Read the model definition and answer for the solid it produces. Units are mm, in the model's axes. A direction names the side the tool comes from. Coordinates: 2 decimals unless noted, no trailing zeros. Loops run counter-clockwise (first coordinate to the right, second up) from the corner with the lowest first, then second, coordinate; pieces in that order, holes last. Notation, with made-up numbers: (-6, -4) - (3, -4) arc R11 cw to (3, 1) - close; hole circle Ø4 at (19.5, 80.5). An arc over 180 degrees is marked (long way). Use one line per item in the form item = value. Start each with the question number.
1) The mould has two halves that part along Y. Classify faces 1 (the face through (-24.43, 9.4, 1.57)), 2 (the face through (10.6, 0.11, 5.67)), 3 (the face through (-3, 0, 3)), 4 (the face through (0.11, -9.43, 9.5)): released by +Y, released by -Y, zero draft, split by the parting line, or undercut.
2) A cutting plane is placed at A-A (x = 0). Give the vertices of the cut face in (y, z).
3) Consider line 1 (X direction, y = 1, z = 3.25); line 2 (Y direction, x = 20, z = 3); line 3 (Z direction, x = -16, y = 0.5). Determine where each line is inside the solid, lowest interval first.
4) Which of the six approach directions +Z, -Z, +X, -X, +Y, -Y give full straight-line access (tool end or side, diameter ignored) to faces 5 (the face through (-9.43, -9.4, 7.61)), 6 (the face through (17, 0, 5.1)), 7 (the face through (17.58, -9.43, 4.5))?
5) A cutting plane is placed at B-B (z = 1). Give the vertices of the cut face in (x, y), and give its area (3 significant figures).
6) Each of these flat-tipped pins is pushed along its axis until it touches: P1, Ø1, axis at x = 9, z = 9, coming from the -Y side; P2, Ø3, axis at x = -1, y = 1, coming from the -Z side; P3, Ø0.8, axis at y = 1, z = 7.5, coming from the +X side; P4, Ø10.5, axis at x = 0, y = 0, coming from the +Z side. Where does it stop, or does it pass through?
7) A cutting plane is placed at D-D (z = 9.25). Give the vertices of the cut face in (x, y), and give its area (3 significant figures).
8) A cutting plane is placed at C-C (y = 0). State how many separate pieces and enclosed holes the cut face has, and give its area (3 significant figures).
from build123d import *

# Parameters (mm, degrees)
F0_W     = 50
F0_H     = 20
F0_R     = 2.25
F0_R_2   = 4
F0_R_3   = 3
F1_DEPTH = 5.1
F2_W     = 20
F2_H     = 20
F2_R     = 3
F2_R_2   = 2.25
F3_DEPTH = 2.5
F4_W     = 20
F4_H     = 20
F4_R     = 4
F5_DEPTH = 2.5
F6_R     = 2


# Not quite as in the source:
# - a feature names something its author has since deleted; it is built from what else it names


with BuildPart() as f1:
    # F0 (on Top) → F1 (new body)
    with BuildSketch(Plane.XY):
        Rectangle(F0_W, F0_H)
        with Locations((-20, 0)):
            Circle(F0_R, mode=Mode.SUBTRACT)
        Circle(F0_R_2, mode=Mode.SUBTRACT)
        with Locations((20, 0)):
            Circle(F0_R, mode=Mode.SUBTRACT)
        Circle(F0_R_2)
        Circle(F0_R_3, mode=Mode.SUBTRACT)
    extrude(amount=F1_DEPTH)

    # F2 (on face) → F3 (join)
    with BuildSketch(Plane.XY.offset(5.1)):
        Rectangle(F2_W, F2_H)
        Circle(F2_R, mode=Mode.SUBTRACT)
        Circle(F2_R)
        Circle(F2_R_2, mode=Mode.SUBTRACT)
    extrude(amount=F3_DEPTH)

    # F4 (on face) → F5 (join)
    with BuildSketch(Plane.XY.offset(7.6)):
        Rectangle(F4_W, F4_H)
        Circle(F4_R, mode=Mode.SUBTRACT)
    extrude(amount=F5_DEPTH)

    # F6
    f6_edges = [f1.edges().sort_by_distance(p)[0] for p in [
        (-25, -10, 2.55),
        (25, -10, 2.55),
        (25, 10, 2.55),
        (25, 0, 5.1),
        (17.5, -10, 5.1),
        (17.5, 10, 5.1),
        (-17.5, -10, 5.1),
        (-25, 0, 5.1),
        (-17.5, 10, 5.1),
        (-25, 10, 2.55),
        (10, -10, 7.6),
        (10, 10, 7.6),
        (-10, -10, 7.6),
        (-10, 10, 7.6),
        (10, 0, 5.1),
        (-10, 0, 5.1),
        (0, -10, 10.1),
        (-10, 0, 10.1),
        (0, 10, 10.1),
        (10, 0, 10.1),
    ]]
    fillet(f6_edges, radius=F6_R)


solid = f1.part
Found:
q1.face_1 = released by +Y
q1.face_2 = zero draft
q1.face_3 = undercut
q1.face_4 = released by -Y
q2.outline = (-10, 0) - (-3, 0) - (-3, 5.1) - (-2.25, 5.1) - (-2.25, 7.6) - (-4, 7.6) - (-4, 10.1) - (-8, 10.1) arc R2 ccw to (-10, 8.1) - close; (2.25, 5.1) - (3, 5.1) - (3, 0) - (10, 0) - (10, 8.1) arc R2 ccw to (8, 10.1) - (4, 10.1) - (4, 7.6) - (2.25, 7.6) - close
q3.line_1 = -24.99 to -22.02, -17.98 to -2.83, 2.83 to 17.98, 22.02 to 24.99
q3.line_2 = -10 to -2.25, 2.25 to 10
q3.line_3 = 0 to 5.1
q4.face_5 = +Z, -X, -Y
q4.face_6 = +Z, +X, +Y, -Y
q4.face_7 = +Z, +X, -Y
q5.outline = (-25, -8) arc R2 ccw to (-23, -10) - (23, -10) arc R2 ccw to (25, -8) - (25, 8) arc R2 ccw to (23, 10) - (-23, 10) arc R2 ccw to (-25, 8) - close; hole circle Ø4.5 at (-20, 0); hole circle Ø6 at (0, 0); hole circle Ø4.5 at (20, 0)
q5.area = 936 mm^2
q6.P1 = -9.81
q6.P2 = 5.1
q6.P3 = 10
q6.P4 = 10.1
q7.outline = (-9.64, -8) arc R1.64 ccw to (-8, -9.64) - (8, -9.64) arc R1.64 ccw to (9.64, -8) - (9.64, 8) arc R1.64 ccw to (8, 9.64) - (-8, 9.64) arc R1.64 ccw to (-9.64, 8) - close; hole circle Ø8 at (0, 0)
q7.area = 319 mm^2
q8.separate_pieces = 4
q8.enclosed_holes = 0
q8.area = 246 mm^2
